Autodesk Inventor part; units mm, degrees
ref_plane "IP1_XY" through (0, 0, 0) normal (1, 0, 0) x (0, 0, -1)
ref_plane "IP1_YZ" through (0, 0, 0) normal (0, 0, -1) x (0, 1, 0)
ref_plane "IP1_ZX" through (0, 0, 0) normal (0, 1, 0) x (1, 0, 0)
sketch "Skizze_2" plane through (0, 0, 0) normal (0, 0, 1) x (1, 0, 0)
  line L0 (12, 0) -> (-0.4283, 0)
  line L1 (-0.4283, 0) -> (-1.15, 1.25)
  line L2 (-1.15, 1.25) -> (-3, 1.25)
  line L3 (-3, 1.25) -> (-3, 2.45)
  arc A0 (-2.7, 2.75) -> (-3, 2.45) centre (-2.7, 2.45) ccw
  line L4 (-2.7, 2.75) -> (0, 2.75)
  line L5 (0, 2.75) -> (0, 1.8)
  arc A1 (0, 1.8) -> (0.0562, 1.7101) centre (0.1, 1.8) ccw
  line L6 (0.0562, 1.7101) -> (0.4662, 1.5101)
  arc A2 (0.4662, 1.5101) -> (0.51, 1.5) centre (0.51, 1.6) ccw
  line L7 (0.51, 1.5) -> (11.6935, 1.5)
  line L8 (11.6935, 1.5) -> (12, 1.1935)
  line L9 (12, 1.1935) -> (12, 0)
  line L10 (12, 0) -> (-0.4283, 0)
revolve "Revolution1" add sketch "Skizze_2" angle 360 about axis through (12, 0, 0) along (1, 0, 0)
thread "Thread1"
sketch "Skizze_1" plane through (-1.15, 0, 0) normal (1, 0, 0) x (0, 0, -1)
  line L0 (-1.25, -0.7217) -> (0, -1.4434)
  line L1 (0, -1.4434) -> (1.25, -0.7217)
  line L2 (1.25, -0.7217) -> (1.25, 0.7217)
  line L3 (1.25, 0.7217) -> (0, 1.4434)
  line L4 (0, 1.4434) -> (-1.25, 0.7217)
  line L5 (-1.25, 0.7217) -> (-1.25, -0.7217)
extrude "Extrusion1" cut sketch "Skizze_1" against normal blind 2.6
ref_plane "IP1_XY" through (0, 0, 0) normal (1, 0, 0) x (0, 0, -1)
ref_plane "IP1_YZ" through (0, 0, 0) normal (0, 0, -1) x (0, 1, 0)
ref_plane "IP1_ZX" through (0, 0, 0) normal (0, 1, 0) x (1, 0, 0)
ref_plane "IP2_XY" through (-3, 0, 0) normal (1, 0, 0) x (0, 0, -1)
ref_plane "IP2_YZ" through (-3, 0, 0) normal (0, 0, -1) x (0, 1, 0)
ref_plane "IP2_ZX" through (-3, 0, 0) normal (0, 1, 0) x (1, 0, 0)
ref_plane "IP3_XY" through (12, 0, 0) normal (1, 0, 0) x (0, 0, -1)
ref_plane "IP3_YZ" through (12, 0, 0) normal (0, 0, -1) x (0, 1, 0)
ref_plane "IP3_ZX" through (12, 0, 0) normal (0, 1, 0) x (1, 0, 0)
ref_plane "IP4_XY" through (0, 0, 0) normal (1, 0, 0) x (0, 0, -1)
ref_plane "IP4_YZ" through (0, 0, 0) normal (0, 0, -1) x (0, 1, 0)
ref_plane "IP4_ZX" through (0, 0, 0) normal (0, 1, 0) x (1, 0, 0)
properties part number "Slotted head cap screw ISO 4762 - M3x12"
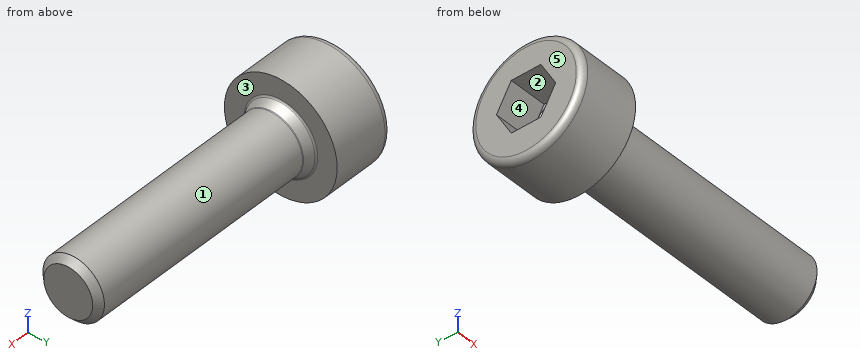
The listing builds one solid part. Answer for the finished solid, in the listing's coordinates (mm). Face numbers are marked on the shaded views. A direction names the side the tool comes from. Give positions to 0.01 mm unless a question says otherwise; leave off trailing zeros. Order: outer loops, then holes, each group sorted by start corner. A loop starts at its lowest first (then second) coordinate and runs counter-clockwise, first axis right, second up. Notation, with made-up numbers: (45, 83.25) -> (89, 83.25) arc R20 ccw to (89, 98.25) -> close; hole circle Ø6 at (48, 8). An arc over 180 degrees is marked (long way). Write each question's results on one line, items separated by ' | '.
Q1. Straight lines are drawn through the part: probe 1 along X at (y, z) = (2, 0.9); probe 2 along Y at (x, z) = (9, -0.05); probe 3 along Y at (x, z) = (-2, 0.7). For each, find the intervals that lie inside material, in ascending order. Write a range as from..to.
Checked values:
probe 1: x = -3..0 | probe 2: y = -1.5..1.5 | probe 3: y = -2.66..-1.04, 1.04..2.66
Q2. The part is cut by section A-A, the plane x = -2. Give the vertices of the cut face in (y, z), and give its area (3 significant figures).
Checked values:
outline: circle Ø5.5 at (0, 0); hole (-1.44, 0) -> (-0.72, -1.25) -> (0.72, -1.25) -> (1.44, 0) -> (0.72, 1.25) -> (-0.72, 1.25) -> close | area: 18.3 mm^2
Q3. This flat-tipped pin is pushed along its axis until it touches: P1, Ø1.2, axis at y = 0.5, z = 0, coming from the -X side. Where does it stop, or does it pass through?
Checked values:
P1: stops at x = -1.06
Q4. Determine the mould class of the marked faces 1, 2 and 3 for opening direction Z: pulls with the +Z half, pulls with the -Z half, needs draft (parallel to the pull), parting line crosses it, or undercut.
Checked values:
face 1: parting line crosses it | face 2: undercut | face 3: needs draft
Q5. The part is cut by section B-B, the plane x = 5. Give the vertices of the cut face in (y, z).
Checked values:
outline: circle Ø3 at (0, 0)
Q6. Which of the six approach directions +Z, -Z, +X, -X, +Y, -Y give full straight-line access (tool end or side, diameter ignored) to the marked faces 4 and 5?
Checked values:
face 4: -X | face 5: +Z, -Z, -X, +Y, -Y
